Model file for the job. Use its own axes, mm. Give positions to 0.01 mm unless a question says otherwise; leave off trailing zeros. Order: outer loops, then holes, each group sorted by start corner. A loop starts at its lowest first (then second) coordinate and runs counter-clockwise, first axis right, second up. Notation, with made-up numbers: (8, -24.75) -> (28, -24.75) arc R21 ccw to (28, -2.75) -> close; hole circle Ø1 at (89, 16). An arc over 180 degrees is marked (long way). Answer in a Markdown table with one row per item. Add a question column.
from build123d import *

# Parameters (mm, degrees)
SM_BASE_FLANGE_2_DEPTH   = 2
SKETCH_26_R              = 2.5
CUT_EXTRUDE_1_DEPTH      = 221.519840377
SKETCH_27_R              = 2.5
CUT_EXTRUDE_2_DEPTH      = 10
SKETCH_28_R              = 2.75
CUT_EXTRUDE_3_DEPTH      = 10
SKETCH_29_R              = 2.75
CUT_EXTRUDE_4_DEPTH      = 10
SKETCH_30_R              = 2.75
CUT_EXTRUDE_5_DEPTH      = 10
MIRROR_3_COPY_1_SKETCH_R = 2.75
MIRROR_3_COPY_1_DEPTH    = 10
SKETCH_31_R              = 2
CUT_EXTRUDE_6_DEPTH      = 10
PATTERN_LINEAR_1_COUNT   = 2
PATTERN_LINEAR_1_PITCH   = 60
SKETCH_32_R              = 2.75
CUT_EXTRUDE_7_DEPTH      = 10
SKETCH_33_R              = 2.75
CUT_EXTRUDE_8_DEPTH      = 10
SKETCH_34_R              = 1.75
CUT_EXTRUDE_9_DEPTH      = 10
SKETCH_35_R              = 2.75
CUT_EXTRUDE_10_DEPTH     = 10
SKETCH_36_R              = 2.75
SKETCH_36_R_2            = 2.5
CUT_EXTRUDE_11_DEPTH     = 10


# Sheet-metal steps are written as plain solids
with BuildPart() as part:
    # 草图2 → 基体-法兰2 (new body)
    with BuildSketch(Plane(origin=(0, 0, 0), x_dir=(1, 0, 0), z_dir=(0, 1, 0))):
        Polygon((-120, 140), (-120, 185), (-95, 185), (-95, 140), (95, 140), (95, 185), (120, 185), (120, 140), (120, -140), (-120, -140), align=None)
    extrude(amount=-SM_BASE_FLANGE_2_DEPTH)

    # 草图26 → 切除-拉伸1 (cut, through all)
    with BuildSketch(Plane(origin=(0, 0, 0), x_dir=(1, 0, 0), z_dir=(0, 1, 0))):
        with Locations(Location((-109, 102, 0), (0, 0, 270))):
            Circle(SKETCH_26_R)
        with Locations(Location((-109, 132, 0), (0, 0, 270))):
            Circle(SKETCH_26_R)
        with Locations(Location((-85, 132, 0), (0, 0, 270))):
            Circle(SKETCH_26_R)
        with Locations(Location((-85, 102, 0), (0, 0, 270))):
            Circle(SKETCH_26_R)
        with Locations(Location((-85, -102, 0), (0, 0, 90))):
            Circle(SKETCH_26_R)
        with Locations(Location((-85, -132, 0), (0, 0, 90))):
            Circle(SKETCH_26_R)
        with Locations(Location((-109, -132, 0), (0, 0, 90))):
            Circle(SKETCH_26_R)
        with Locations(Location((-109, -102, 0), (0, 0, 90))):
            Circle(SKETCH_26_R)
        with Locations(Location((85, 102, 0), (0, 0, 90))):
            Circle(SKETCH_26_R)
        with Locations(Location((85, 132, 0), (0, 0, 90))):
            Circle(SKETCH_26_R)
        with Locations(Location((109, 132, 0), (0, 0, 90))):
            Circle(SKETCH_26_R)
        with Locations(Location((109, 102, 0), (0, 0, 90))):
            Circle(SKETCH_26_R)
        with Locations(Location((109, -102, 0), (0, 0, 270))):
            Circle(SKETCH_26_R)
        with Locations(Location((109, -132, 0), (0, 0, 270))):
            Circle(SKETCH_26_R)
        with Locations(Location((85, -132, 0), (0, 0, 270))):
            Circle(SKETCH_26_R)
        with Locations(Location((85, -102, 0), (0, 0, 270))):
            Circle(SKETCH_26_R)
    extrude(amount=-CUT_EXTRUDE_1_DEPTH, mode=Mode.SUBTRACT)

    # 草图27 → 切除-拉伸2 (cut)
    with BuildSketch(Plane.XZ.offset(2)):
        with Locations(Location((-35.355339059, 35.355339059, 0), (0, 0, 270))):
            Circle(SKETCH_27_R)
        with Locations(Location((35.355339059, 35.355339059, 0), (0, 0, 270))):
            Circle(SKETCH_27_R)
        with Locations(Location((35.355339059, -35.355339059, 0), (0, 0, 270))):
            Circle(SKETCH_27_R)
        with Locations(Location((-35.355339059, -35.355339059, 0), (0, 0, 270))):
            Circle(SKETCH_27_R)
    extrude(amount=-CUT_EXTRUDE_2_DEPTH, mode=Mode.SUBTRACT)

    # 草图28 → 切除-拉伸3 (cut)
    with BuildSketch(Plane.XZ.offset(2)):
        with Locations(Location((-60, -80, 0), (0, 0, 270))):
            Circle(SKETCH_28_R)
        with Locations(Location((-37.250025969, -92.803208809, 0), (0, 0, 270))):
            Circle(SKETCH_28_R)
        with Locations(Location((-78.661073186, -61.744923397, 0), (0, 0, 270))):
            Circle(SKETCH_28_R)
        with Locations(Location((78.661073186, -61.744923397, 0), (0, 0, 90))):
            Circle(SKETCH_28_R)
        with Locations(Location((37.250025969, -92.803208809, 0), (0, 0, 90))):
            Circle(SKETCH_28_R)
        with Locations(Location((60, -80, 0), (0, 0, 90))):
            Circle(SKETCH_28_R)
        with Locations(Location((-78.661073186, 61.744923397, 0), (0, 0, 90))):
            Circle(SKETCH_28_R)
        with Locations(Location((-37.250025969, 92.803208809, 0), (0, 0, 90))):
            Circle(SKETCH_28_R)
        with Locations(Location((-60, 80, 0), (0, 0, 90))):
            Circle(SKETCH_28_R)
        with Locations(Location((60, 80, 0), (0, 0, 270))):
            Circle(SKETCH_28_R)
        with Locations(Location((37.250025969, 92.803208809, 0), (0, 0, 270))):
            Circle(SKETCH_28_R)
        with Locations(Location((78.661073186, 61.744923397, 0), (0, 0, 270))):
            Circle(SKETCH_28_R)
    extrude(amount=-CUT_EXTRUDE_3_DEPTH, mode=Mode.SUBTRACT)

    # 草图29 → 切除-拉伸4 (cut)
    with BuildSketch(Plane.XZ.offset(2)):
        with Locations(Location((105, -175, 0), (0, 0, 270))):
            Circle(SKETCH_29_R)
        with Locations(Location((105, -156, 0), (0, 0, 270))):
            Circle(SKETCH_29_R)
        with Locations(Location((105, -145, 0), (0, 0, 270))):
            Circle(SKETCH_29_R)
    cut_extrude_4 = extrude(amount=-CUT_EXTRUDE_4_DEPTH, mode=Mode.SUBTRACT)

    # 镜向1: 切除-拉伸4 across plane
    add(cut_extrude_4.mirror(Plane(origin=(0, 0, 0), x_dir=(0, 0, 1), z_dir=(1, 0, 0))), mode=Mode.SUBTRACT)

    # 草图30 → 切除-拉伸5 (cut)
    with BuildSketch(Plane(origin=(0, 0, 0), x_dir=(1, 0, 0), z_dir=(0, 1, 0))):
        with Locations(Location((-92, 90.5, 0), (0, 0, 270))):
            Circle(SKETCH_30_R)
        with Locations(Location((-92, 79.5, 0), (0, 0, 270))):
            Circle(SKETCH_30_R)
        with Locations(Location((-72, 79.5, 0), (0, 0, 270))):
            Circle(SKETCH_30_R)
        with Locations(Location((-72, 90.5, 0), (0, 0, 270))):
            Circle(SKETCH_30_R)
    cut_extrude_5 = extrude(amount=-CUT_EXTRUDE_5_DEPTH, mode=Mode.SUBTRACT)

    # 镜向2: 切除-拉伸5 across plane
    add(cut_extrude_5.mirror(Plane.XY), mode=Mode.SUBTRACT)

    # 镜向3: 切除-拉伸5 across plane
    add(cut_extrude_5.mirror(Plane(origin=(0, 0, 0), x_dir=(0, 0, 1), z_dir=(1, 0, 0))), mode=Mode.SUBTRACT)

    # 镜向3 copy 1 sketch → 镜向3 copy 1 (cut)
    with BuildSketch(Plane(origin=(0, 0, 0), x_dir=(-1, 0, 0), z_dir=(0, 1, 0))):
        with Locations(Location((-92, 90.5, 0), (0, 0, 270))):
            Circle(MIRROR_3_COPY_1_SKETCH_R)
        with Locations(Location((-92, 79.5, 0), (0, 0, 270))):
            Circle(MIRROR_3_COPY_1_SKETCH_R)
        with Locations(Location((-72, 79.5, 0), (0, 0, 270))):
            Circle(MIRROR_3_COPY_1_SKETCH_R)
        with Locations(Location((-72, 90.5, 0), (0, 0, 270))):
            Circle(MIRROR_3_COPY_1_SKETCH_R)
    extrude(amount=-MIRROR_3_COPY_1_DEPTH, mode=Mode.SUBTRACT)

    # 草图31 → 切除-拉伸6 (cut)
    with BuildSketch(Plane(origin=(0, 0, 0), x_dir=(1, 0, 0), z_dir=(0, 1, 0))):
        with Locations(Location((31.05, -52, 0), (0, 0, 270))):
            Circle(SKETCH_31_R)
        with Locations(Location((31.05, -7.74, 0), (0, 0, 270))):
            Circle(SKETCH_31_R)
        with Locations(Location((100, -7.74, 0), (0, 0, 270))):
            Circle(SKETCH_31_R)
        with Locations(Location((100, -52, 0), (0, 0, 270))):
            Circle(SKETCH_31_R)
    cut_extrude_6 = extrude(amount=-CUT_EXTRUDE_6_DEPTH, mode=Mode.SUBTRACT)

    # 阵列(线性)1: 切除-拉伸6 ×2
    with Locations(*[(0, 0, -i * PATTERN_LINEAR_1_PITCH) for i in range(1, PATTERN_LINEAR_1_COUNT)]):
        add(cut_extrude_6, mode=Mode.SUBTRACT)

    # 草图32 → 切除-拉伸7 (cut)
    with BuildSketch(Plane(origin=(0, 0, 0), x_dir=(1, 0, 0), z_dir=(0, 1, 0))):
        with Locations(Location((-20, 77.5, 0), (0, 0, 270))):
            Circle(SKETCH_32_R)
        with Locations(Location((-20, 11.8, 0), (0, 0, 270))):
            Circle(SKETCH_32_R)
    extrude(amount=-CUT_EXTRUDE_7_DEPTH, mode=Mode.SUBTRACT)

    # 草图33 → 切除-拉伸8 (cut)
    with BuildSketch(Plane(origin=(0, 0, 0), x_dir=(1, 0, 0), z_dir=(0, 1, 0))):
        with Locations(Location((-70, -52.5, 0), (0, 0, 270))):
            Circle(SKETCH_33_R)
        with Locations(Location((-70, 4.5, 0), (0, 0, 270))):
            Circle(SKETCH_33_R)
        with Locations(Location((-40, 4.5, 0), (0, 0, 270))):
            Circle(SKETCH_33_R)
        with Locations(Location((-40, -52.5, 0), (0, 0, 270))):
            Circle(SKETCH_33_R)
    extrude(amount=-CUT_EXTRUDE_8_DEPTH, mode=Mode.SUBTRACT)

    # 草图34 → 切除-拉伸9 (cut)
    with BuildSketch(Plane(origin=(0, 0, 0), x_dir=(1, 0, 0), z_dir=(0, 1, 0))):
        with Locations(Location((15, -95, 0), (0, 0, 270))):
            Circle(SKETCH_34_R)
        with Locations(Location((15, -64, 0), (0, 0, 270))):
            Circle(SKETCH_34_R)
        with Locations(Location((-46, -64, 0), (0, 0, 270))):
            Circle(SKETCH_34_R)
        with Locations(Location((-46, -95, 0), (0, 0, 270))):
            Circle(SKETCH_34_R)
    extrude(amount=-CUT_EXTRUDE_9_DEPTH, mode=Mode.SUBTRACT)

    # 草图35 → 切除-拉伸10 (cut)
    with BuildSketch(Plane.XZ.offset(2)):
        with Locations(Location((30, -126, 0), (0, 0, 270))):
            Circle(SKETCH_35_R)
        with Locations(Location((-30, -126, 0), (0, 0, 90))):
            Circle(SKETCH_35_R)
    extrude(amount=-CUT_EXTRUDE_10_DEPTH, mode=Mode.SUBTRACT)

    # 草图36 → 切除-拉伸11 (cut)
    with BuildSketch(Plane.XZ.offset(2)):
        with Locations(Location((-114, -15, 0), (0, 0, 270))):
            Circle(SKETCH_36_R)
        with Locations(Location((-114, 15, 0), (0, 0, 90))):
            Circle(SKETCH_36_R)
        with Locations(Location((114, -15, 0), (0, 0, 90))):
            Circle(SKETCH_36_R)
        with Locations(Location((114, 15, 0), (0, 0, 270))):
            Circle(SKETCH_36_R)
        with Locations(Location((15, 134, 0), (0, 0, 90))):
            Circle(SKETCH_36_R_2)
        with Locations(Location((-15, 134, 0), (0, 0, 270))):
            Circle(SKETCH_36_R_2)
        with Locations(Location((15, -121, 0), (0, 0, 270))):
            Circle(SKETCH_36_R)
        with Locations(Location((-15, -121, 0), (0, 0, 90))):
            Circle(SKETCH_36_R)
    extrude(amount=-CUT_EXTRUDE_11_DEPTH, mode=Mode.SUBTRACT)


solid = part.part
Item 1: Pin check, flat tip, straight feed: pin 1 Ø1 at (x, z) = (28, -118) entering from +Y. Stop position of the tip, or through.
Item 2: Saw through at B-B on y = -1.55. Give the number of separate pieces and of enclosed holes in the cut face, plus the area to 3 significant figures.
Item 3: Saw through at A-A on x = -9. List the corners of the cut face in (y, z).
Item 4: Wall check: line 1 (X direction, y = -1.45, z = -156); line 2 (X direction, y = -1, z = -132); line 3 (X direction, y = -0.7, z = -8). Give the ranges that are in metal, low to high.
Evaluation:
| question | item | result |
|---|---|---|
| 1 | pin 1 | stops at y = 0 |
| 2 | separate pieces | 1 |
| 2 | enclosed holes | 82 |
| 2 | area | 67,700 mm2 |
| 3 | outline | (-2, -140) -> (0, -140) -> (0, 140) -> (-2, 140) -> close |
| 4 | line 1 | x = -120 to -107.75, -102.25 to -95, 95 to 102.25, 107.75 to 120 |
| 4 | line 2 | x = -120 to -111.5, -106.5 to -87.5, -82.5 to 82.5, 87.5 to 106.5, 111.5 to 120 |
| 4 | line 3 | x = -120 to 29.05, 33.05 to 98, 102 to 120 |
